The model under review builds one solid part; all positions refer to its coordinate system, in mm. Round coordinates to 2 decimals unless told otherwise and drop trailing zeros. Write each loop counter-clockwise with the first axis right and the second up, starting at its lowest first coordinate (ties: lowest second). Pieces come first, ordered by that corner, then holes. Notation, with made-up numbers: M 1.5,1 L 22.5,1 A26 ccw 22.5,34 Z; hole C 60,8.5 d4. An arc over 180 degrees is marked long. One line per item, written item: value. Start each with the question number.
1) Take a section at B-B, the plane z = 4.25. Write out the cut boundary in (x, y), and give its area (3 significant figures).
2) Take a section at C-C, the plane x = 10. Write out the cut boundary in (y, z).
3) Mouldability with a two-part tool opening along X and no side actions: class faces 1 (the face through (11.18, -14.92, 3.13)), 2 (the face through (55, -9, 3)), 3 (the face through (0, -9, 3)) as +X half, -X half, draft (parallel to the pull), parting line (faces both ways), or undercut.
4) Wall thickness on probe 1 along Y at (x, z) = (10, 2); probe 2 along X at (y, z) = (-15.5, 5.75); probe 3 along X at (y, z) = (-15.75, 1): over which ranges is each line inside the solid? List them lowest first.
5) Take a section at A-A, the plane y = -16. Write out the cut boundary in (x, z), and give its area (3 significant figures).
6) For P1, Ø3, axis at x = 10, y = -16, coming from the -Z side, flat-tipped, find the tip position at first contact; note if it passes through.
7) Take a section at D-D, the plane y = -18.5. Write out the cut boundary in (x, z).
from build123d import *

# Parameters (mm, degrees)
SKETCH1_W             = 55
SKETCH1_H             = 20
BOSS_EXTRUDE1_DEPTH   = 6.35
F_3_0MM_DOWEL_HOLE1_D = 3.2
CHAMFER1_SIZE         = 3


with BuildPart() as part:
    # Sketch1 → Boss-Extrude1 (new body)
    with BuildSketch(Plane.XY):
        with Locations((27.5, -10)):
            Rectangle(SKETCH1_W, SKETCH1_H)
    extrude(amount=BOSS_EXTRUDE1_DEPTH)

    # Ø3.0mm Dowel Hole1 (through all)
    with Locations(Plane.XY.offset(6.35)):
        with Locations((10, -16), (45, -16)):
            Hole(F_3_0MM_DOWEL_HOLE1_D / 2)

    # Chamfer1
    chamfer1_edges = [part.edges().sort_by_distance(p)[0] for p in [
        (55, -20, 3.175),
        (0, -20, 3.175),
    ]]
    chamfer(chamfer1_edges, length=CHAMFER1_SIZE)


solid = part.part
Checked values:
1. outline: M 0,-17 L 3,-20 L 52,-20 L 55,-17 L 55,0 L 0,0 Z; hole C 10,-16 d3.2; hole C 45,-16 d3.2
1. area: 1,070 mm2
2. outline: M -20,0 L -17.6,0 L -17.6,6.35 L -20,6.35 Z; M -14.4,0 L 0,0 L 0,6.35 L -14.4,6.35 Z
3. face 1: undercut
3. face 2: +X half
3. face 3: -X half
4. probe 1: y = -20 to -17.6, -14.4 to 0
4. probe 2: x = 0 to 8.48, 11.52 to 43.48, 46.52 to 55
4. probe 3: x = 0 to 8.42, 11.58 to 43.42, 46.58 to 55
5. outline: M 0,0 L 8.4,0 L 8.4,6.35 L 0,6.35 Z; M 11.6,0 L 43.4,0 L 43.4,6.35 L 11.6,6.35 Z; M 46.6,0 L 55,0 L 55,6.35 L 46.6,6.35 Z
5. area: 309 mm2
6. P1: passes through
7. outline: M 1.5,0 L 53.5,0 L 53.5,6.35 L 1.5,6.35 Z
